Geometry check sheet. Reference: drawing and pictorial views, mm from the part's lowest x, y, z. Round coordinates to 2 decimals unless told otherwise and drop trailing zeros. Loops run counter-clockwise (first coordinate to the right, second up) from the corner with the lowest first, then second, coordinate; pieces in that order, holes last. Notation, with made-up numbers: (-22, 47.25) -> (8, 47.25) arc R16 ccw to (8, 63.25) -> close; hole circle Ø7 at (26.25, 40). An arc over 180 degrees is marked (long way). Write item = value, one per line.
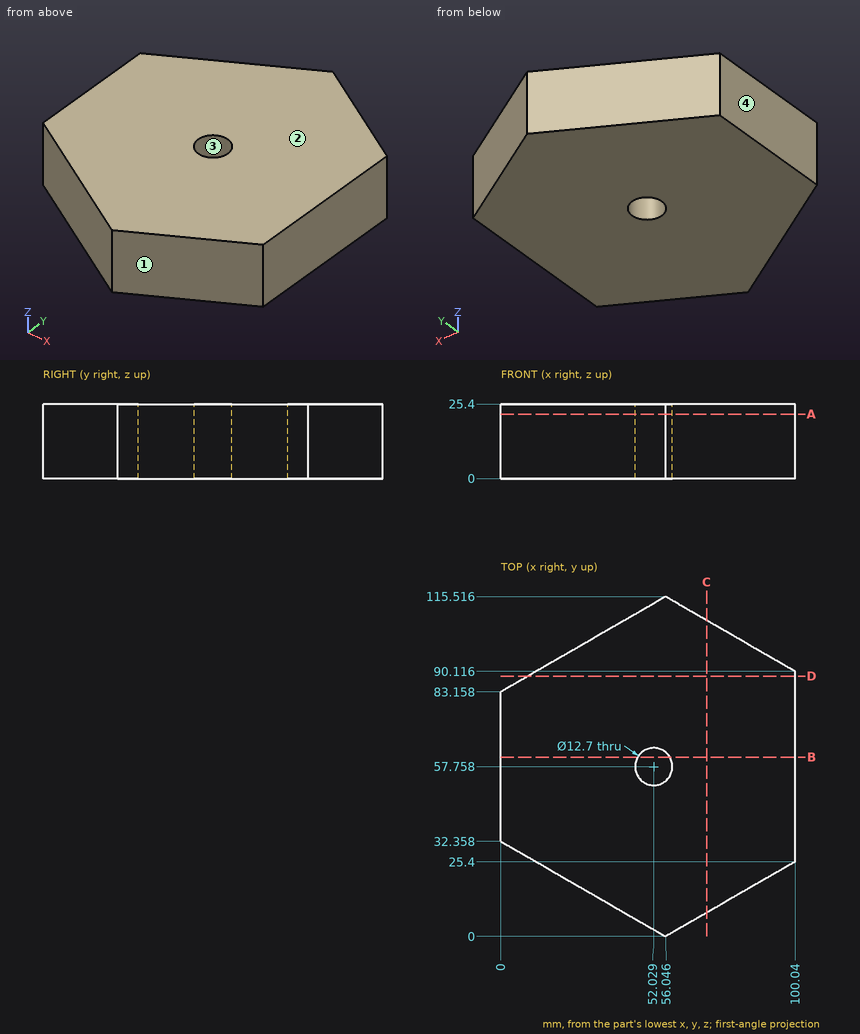
(1) Sectioned sample at D-D, the plane y = 88.5. Record the cut outline in (x, z), and give its area (3 significant figures).
Filled sheet:
outline = (9.25, 0) -> (100.04, 0) -> (100.04, 25.4) -> (9.25, 25.4) -> close
area = 2,310 mm2
(2) Sectioned sample at C-C, the plane x = 70. Record the cut outline in (y, z), and give its area (4 significant figures).
Filled sheet:
outline = (8.06, 0) -> (107.46, 0) -> (107.46, 25.4) -> (8.06, 25.4) -> close
area = 2,525 mm2
(3) Sectioned sample at A-A, the plane z = 22. Record the cut outline in (x, y).
Filled sheet:
outline = (0, 32.36) -> (56.05, 0) -> (100.04, 25.4) -> (100.04, 90.12) -> (56.05, 115.52) -> (0, 83.16) -> close; hole circle Ø12.7 at (52.03, 57.76)
(4) Draft check along X on the marked faces 1, 2, 3 and 4. Enter one of: released by +X, released by -X, zero draft, split by the parting line, or undercut.
Filled sheet:
face_1 = released by +X
face_2 = zero draft
face_3 = undercut
face_4 = released by -X
(5) Material ranges on probe 1 along Y at (x, z) = (47, 23.5) (1 decimal); probe 2 along X at (y, z) = (52.5, 14); probe 3 along X at (y, z) = (53, 14.75) (1 decimal), recorded low to high. Write a range as from..to.
Filled sheet:
probe_1 = 5.2..53.9, 61.6..110.3
probe_2 = 0..48.47, 55.59..100.04
probe_3 = 0..47.8, 56.2..100
(6) Sectioned sample at B-B, the plane y = 61. Record the cut outline in (x, z).
Filled sheet:
outline = (0, 0) -> (46.57, 0) -> (46.57, 25.4) -> (0, 25.4) -> close; (57.49, 0) -> (100.04, 0) -> (100.04, 25.4) -> (57.49, 25.4) -> close
(7) Go/stop test with a flat-tipped pin: pin 1 Ø10 at (x, y) = (52.03, 57.76) entering from +Z. Record where the tip stops, or that it passes through.
Filled sheet:
pin_1 = through
